from build123d import *

# Parameters (mm, degrees)
ENCLOSURE_TOP_SKETCH_W          = 76
ENCLOSURE_TOP_SKETCH_H          = 54
ENCLOSURE_TOP_FEATURE_DEPTH     = 4
SCREW_HOLES_SKETCH_R            = 1.6
SCREW_HOLES_FEATURE_DEPTH       = 5
CAMERA_LIGHT_HOLE_SKETCH_R      = 7.5
CAMERA_LIGHT_HOLE_SKETCH_W      = 20
CAMERA_LIGHT_HOLE_SKETCH_H      = 16
CAMERA_LIGHT_HOLE_SKETCH_W_2    = 10
CAMERA_LIGHT_HOLE_SKETCH_H_2    = 15
CAMERA_LIGHT_HOLE_SKETCH_W_3    = 12
CAMERA_LIGHT_HOLE_SKETCH_H_3    = 12
CAMERA_LIGHT_HOLE_FEATURE_DEPTH = 5
FILTER_COVER_SKETCH_R           = 9
FILTER_COVER_FEATURE_DEPTH      = 3.5
FILTER_HOLE_SKETCH_R            = 6.5
FILTER_HOLE_CUT_DEPTH           = 3.5
FILLET6_R                       = 1.5
FILLET7_R                       = 1
FILLET8_R                       = 1
FILLET9_R                       = 1
FILLET10_R                      = 1
FILLET11_R                      = 1


with BuildPart() as part:
    # Enclosure Top Sketch → Enclosure Top Feature (new body)
    with BuildSketch(Plane.XY):
        Rectangle(ENCLOSURE_TOP_SKETCH_W, ENCLOSURE_TOP_SKETCH_H)
    extrude(amount=ENCLOSURE_TOP_FEATURE_DEPTH)

    # Screw Holes Sketch → Screw Holes Feature (cut, through all)
    with BuildSketch(Plane.XY.offset(4)):
        with Locations((-31.1, 20.5)):
            Circle(SCREW_HOLES_SKETCH_R)
        with Locations((31.1, 20.5)):
            Circle(SCREW_HOLES_SKETCH_R)
        with Locations((31.1, -20.5)):
            Circle(SCREW_HOLES_SKETCH_R)
        with Locations((-31.1, -20.5)):
            Circle(SCREW_HOLES_SKETCH_R)
    extrude(amount=-SCREW_HOLES_FEATURE_DEPTH, mode=Mode.SUBTRACT)

    # Camera + Light Hole Sketch → Camera _ Light Hole Feature (cut, through all)
    with BuildSketch(Plane.XY.offset(4)):
        with Locations((-13, -1)):
            Circle(CAMERA_LIGHT_HOLE_SKETCH_R)
        with Locations((9, -1)):
            Rectangle(CAMERA_LIGHT_HOLE_SKETCH_W, CAMERA_LIGHT_HOLE_SKETCH_H)
        with Locations((33, -1)):
            Rectangle(CAMERA_LIGHT_HOLE_SKETCH_W_2, CAMERA_LIGHT_HOLE_SKETCH_H_2)
        with Locations((22.5, 18.714)):
            Rectangle(CAMERA_LIGHT_HOLE_SKETCH_W_3, CAMERA_LIGHT_HOLE_SKETCH_H_3)
    extrude(amount=-CAMERA_LIGHT_HOLE_FEATURE_DEPTH, mode=Mode.SUBTRACT)

    # Filter Cover Sketch → Filter Cover Feature (add)
    with BuildSketch(Plane(origin=(0, 0, 4), x_dir=(-1, 0, 0), z_dir=(0, 0, -1))):
        with Locations((12, 0)):
            Circle(FILTER_COVER_SKETCH_R)
    extrude(amount=-FILTER_COVER_FEATURE_DEPTH)

    # Filter Hole Sketch → Filter Hole Cut (cut)
    with BuildSketch(Plane.XY.offset(4)):
        with Locations((-12, 0)):
            Circle(FILTER_HOLE_SKETCH_R)
    extrude(amount=FILTER_HOLE_CUT_DEPTH, mode=Mode.SUBTRACT)

    # Fillet6
    fillet6_edges = [part.edges().sort_by_distance(p)[0] for p in [
        (-3, 0, 7.5),
    ]]
    fillet(fillet6_edges, radius=FILLET6_R)

    # Fillet7
    fillet7_edges = [part.edges().sort_by_distance(p)[0] for p in [
        (0, 27, 4),
    ]]
    fillet(fillet7_edges, radius=FILLET7_R)

    # Fillet8
    fillet8_edges = [part.edges().sort_by_distance(p)[0] for p in [
        (0, -27, 4),
    ]]
    fillet(fillet8_edges, radius=FILLET8_R)

    # Fillet9
    fillet9_edges = [part.edges().sort_by_distance(p)[0] for p in [
        (-38, 0, 4),
        (-38, 27, 1.5),
        (-38, 26.707106781, 3.707106781),
        (-38, -27, 1.5),
        (-38, -26.707106781, 3.707106781),
    ]]
    fillet(fillet9_edges, radius=FILLET9_R)

    # Fillet10
    fillet10_edges = [part.edges().sort_by_distance(p)[0] for p in [
        (38, 27, 1.5),
        (38, 26.707106781, 3.707106781),
        (38, 16.25, 4),
    ]]
    fillet(fillet10_edges, radius=FILLET10_R)

    # Fillet11
    fillet11_edges = [part.edges().sort_by_distance(p)[0] for p in [
        (38, -17.25, 4),
        (38, -27, 1.5),
        (38, -26.707106781, 3.707106781),
    ]]
    fillet(fillet11_edges, radius=FILLET11_R)


solid = part.part
Input: part model. Units: mm. Frame: model coordinates. A direction names the side the tool comes from. Give positions to 0.01 mm unless a question says otherwise; leave off trailing zeros. Write each loop counter-clockwise with the first axis right and the second up, starting at its lowest first coordinate (ties: lowest second). Pieces come first, ordered by that corner, then holes.
Q1. First-contact query: P1, Ø2, axis at y = 0, z = 2, coming from the +X side; P2, Ø2, axis at x = -10, y = 2.5, coming from the +Z side; P3, Ø3, axis at x = -27, y = -5, coming from the +Z side. Flat tips, straight axial feed; report the tip coordinate or a pass-through.
Q2. Section B-B, the plane x = 12.5. Output: boundary loops of the cut face in (y, z), plus the area to 3 significant figures.
Q3. Pull-direction query (Y, two-part tool) for faces 1 (the face through (-1, -27, 1)), 2 (the face through (38, -17, 1)), 3 (the face through (22, 24.714, 2)); classes: pulls with the +Y half, pulls with the -Y half, needs draft (parallel to the pull), parting line crosses it, or undercut.
Q4. Section D-D, the plane y = 18. Output: boundary loops of the cut face in (x, z).
Q5. Section A-A, the plane y = -20.5. Output: boundary loops of the cut face in (x, z).
Q6. Material intervals for probe 1 along Y at (x, z) = (-31.1, 0.9); probe 2 along Y at (x, z) = (18.5, 2); probe 3 along Y at (x, z) = (-13, 2.1), sorted ascending.
Q7. Set-up query: faces 4 (the face through (-5.8, 1.95, 5.73)), 5 (the face through (38, 16, 1)), 6 (the face through (33, 6.5, 2)), 7 (the face through (22, 12.714, 2)), 8 (the face through (-18.5, 4.1, 2)). Return all of +Z, -Z, +X, -X, +Y, -Y with unobstructed straight access to the full face (end or side cutting, diameter ignored); none if empty.
Q8. Section C-C, the plane x = -31.1. Output: boundary loops of the cut face in (y, z).
Filled in:
1. P1: stops at x = 28
1. P2: passes through
1. P3: stops at z = 4
2. outline: (-27, 0) - (-9, 0) - (-9, 4) - (-26, 4) arc R1 ccw to (-27, 3) - close; (7, 0) - (27, 0) - (27, 3) arc R1 ccw to (26, 4) - (7, 4) - close
2. area: 152 mm2
3. face 1: pulls with the -Y half
3. face 2: needs draft
3. face 3: undercut
4. outline: (-38, 0) - (16.5, 0) - (16.5, 4) - (-37, 4) arc R1 ccw to (-38, 3) - close; (28.5, 0) - (38, 0) - (38, 3) arc R1 ccw to (37, 4) - (28.5, 4) - close
5. outline: (-38, 0) - (-32.7, 0) - (-32.7, 4) - (-37, 4) arc R1 ccw to (-38, 3) - close; (-29.5, 0) - (29.5, 0) - (29.5, 4) - (-29.5, 4) - close; (32.7, 0) - (38, 0) - (38, 3) arc R1 ccw to (37, 4) - (32.7, 4) - close
6. probe 1: y = -27 to -22.1, -18.9 to 18.9, 22.1 to 27
6. probe 2: y = -27 to -9, 7 to 12.71, 24.71 to 27
6. probe 3: y = -27 to -8.5, 6.5 to 27
7. face 4: +Z
7. face 5: +Z, -Z, +X, +Y, -Y
7. face 6: +Z, -Z, +X
7. face 7: +Z, -Z
7. face 8: -Z
8. outline: (-27, 0) - (-22.1, 0) - (-22.1, 4) - (-26, 4) arc R1 ccw to (-27, 3) - close; (-18.9, 0) - (18.9, 0) - (18.9, 4) - (-18.9, 4) - close; (22.1, 0) - (27, 0) - (27, 3) arc R1 ccw to (26, 4) - (22.1, 4) - close
